from build123d import *

# Parameters (mm, degrees)
ESQUISSE1_W             = 149
ESQUISSE1_H             = 10
BOSS_EXTRU_1_DEPTH      = 3
ESQUISSE2_R             = 1.005
ESQUISSE2_W             = 7
ESQUISSE2_H             = 3
ENL_V_MAT_EXTRU_1_DEPTH = 150.365323954


with BuildPart() as part:
    # Esquisse1 → Boss.-Extru.1 (new body)
    with BuildSketch(Plane.XY):
        with Locations((74.5, 5)):
            Rectangle(ESQUISSE1_W, ESQUISSE1_H)
    extrude(amount=BOSS_EXTRU_1_DEPTH)

    # Esquisse2 → Enlèv. mat.-Extru.1 (cut, through all)
    with BuildSketch(Plane(origin=(0, 0, 0), x_dir=(-1, 0, 0), z_dir=(0, 0, -1))):
        with Locations((-3, 3)):
            Circle(ESQUISSE2_R)
        with Locations((-146, 3)):
            Circle(ESQUISSE2_R)
        with Locations((-140.5, 6.5)):
            Rectangle(ESQUISSE2_W, ESQUISSE2_H)
        with Locations((-126.5, 6.5)):
            Rectangle(ESQUISSE2_W, ESQUISSE2_H)
        with Locations((-112.5, 6.5)):
            Rectangle(ESQUISSE2_W, ESQUISSE2_H)
        with Locations((-98.5, 6.5)):
            Rectangle(ESQUISSE2_W, ESQUISSE2_H)
        with Locations((-84.5, 6.5)):
            Rectangle(ESQUISSE2_W, ESQUISSE2_H)
        with Locations((-70.5, 6.5)):
            Rectangle(ESQUISSE2_W, ESQUISSE2_H)
        with Locations((-56.5, 6.5)):
            Rectangle(ESQUISSE2_W, ESQUISSE2_H)
        with Locations((-42.5, 6.5)):
            Rectangle(ESQUISSE2_W, ESQUISSE2_H)
        with Locations((-28.5, 6.5)):
            Rectangle(ESQUISSE2_W, ESQUISSE2_H)
        with Locations((-14.5, 6.5)):
            Rectangle(ESQUISSE2_W, ESQUISSE2_H)
    extrude(amount=-ENL_V_MAT_EXTRU_1_DEPTH, mode=Mode.SUBTRACT)


solid = part.part
Can you work these out from the model? Positions are in its coordinate system, mm. A direction names the side the tool comes from. Coordinates: 2 decimals unless noted, no trailing zeros. Write each loop counter-clockwise with the first axis right and the second up, starting at its lowest first coordinate (ties: lowest second). Pieces come first, ordered by that corner, then holes.
Q1. Imagine slicing it at A-A, the plane x = 14.5. List the corners of the cut face in (y, z) for me.
Results found:
outline: (0, 0) - (5, 0) - (5, 3) - (0, 3) - close; (8, 0) - (10, 0) - (10, 3) - (8, 3) - close
Q2. Which directions (+Z, -Z, +X, -X, +Y, -Y) give clear straight access to the entire face, cutting with the end or side of a thin tool? Please do faces 1 (the face through (0, 5, 1)), 2 (the face through (123, 6, 1)).
Results found:
face 1: +Z, -Z, -X, +Y, -Y
face 2: +Z, -Z
Q3. Imagine slicing it at B-B, the plane z = 0.45. Count the separate pieces of the cut face and the enclosed holes in it, plus the area to 3 significant figures.
Results found:
separate pieces: 1
enclosed holes: 12
area: 1,270 mm2
Q4. For P1, Ø1.5, axis at x = 55, z = 1, coming from the -Y side, with a flat end and sliding along its axis, tell me the tip position at first contact or that it passes through.
Results found:
P1: stops at y = 0
Q5. Please list where these lines run through material, in increasing order: L1, parallel to X at y = 2.5, z = 1.9; L2, parallel to Y at x = 3, z = 2.1 (3 decimals); L3, parallel to Y at x = 11.5, z = 2.2.
Results found:
L1: x = 0 to 2.13, 3.87 to 145.13, 146.87 to 149
L2: y = 0 to 1.995, 4.005 to 10
L3: y = 0 to 5, 8 to 10
Q6. If we mould it in two halves opening along Y, with no side actions, what happens to faces 3 (the face through (130, 6, 1)), 4 (the face through (73, 4, 0))? For each: +Y half, -Y half, draft (parallel to the pull), parting line (faces both ways), or undercut.
Results found:
face 3: undercut
face 4: draft
